```python
from build123d import *

# Parameters (mm, degrees)
F0_R     = 47.625
F0_R_2   = 38.1
F1_DEPTH = 15.24
F2_R     = 47.625
F2_R_2   = 41.275
F3_DEPTH = 12.065
F4_SIZE2 = 6.34999
F4_SIZE  = 2.53999


# Not quite as in the source:
# - a fillet or chamfer is up to 0.001 mm smaller than in the source, because OpenCascade refuses the exact size


with BuildPart() as f1:
    # F0 (on Front) → F1 (new body)
    with BuildSketch(Plane.XZ):
        Circle(F0_R)
        Circle(F0_R_2, mode=Mode.SUBTRACT)
    extrude(amount=F1_DEPTH)

    # F2 (on face) → F3 (cut)
    with BuildSketch(Plane.XZ.offset(15.24)):
        Circle(F2_R)
        Circle(F2_R_2, mode=Mode.SUBTRACT)
    extrude(amount=-F3_DEPTH, mode=Mode.SUBTRACT)

    # F4 (size 2.54 and 6.35 in the source; OpenCascade refuses exactly that, so slightly less here)
    f4_edges = [f1.edges().sort_by_distance(p)[0] for p in [
        (-41.275, -3.175, 0),
    ]]
    f4_side = f1.faces().sort_by_distance((-41.275, -9.2075, 0))[0]
    chamfer(f4_edges, length=F4_SIZE, length2=F4_SIZE2, reference=f4_side)


solid = f1.part
```
Geometry check sheet. Reference: the model listing, model coordinates, mm. A direction names the side the tool comes from. Coordinates: 2 decimals unless noted, no trailing zeros. Write each loop counter-clockwise with the first axis right and the second up, starting at its lowest first coordinate (ties: lowest second). Pieces come first, ordered by that corner, then holes. Notation, with made-up numbers: M 11,-19 L 19,-19 A19 cw 19,14 Z; hole C -16,49 d1. An arc over 180 degrees is marked long. Use one line per item in the form item = value. Start each with the question number.
1) Thickness scan on probe 1 along Z at (x, y) = (0, -10.75) (3 decimals); probe 2 along X at (y, z) = (-12, -25); probe 3 along X at (y, z) = (-7.25, -2.5). Record the ranges inside material, lowest first. Write a range as from..to.
2) Section check C-C on y = -9.75. Enter the section's corners in (x, z) (3 decimals), and give its area (3 significant figures).
3) Go/stop test with flat-tipped pins: pin 1 Ø6 at (x, y) = (-6, -5.5) entering from -Z; pin 2 Ø6 at (x, y) = (-21, -11.5) entering from +Z; pin 3 Ø3 at (x, y) = (-35.5, -12) entering from +Z. Record where each tip stops, or that it passes through.
4) Release check for a two-part mould opening along X. For faces 1 (the cylindrical face through (-37.794, -1.565, -28.979)), 2 (the cylindrical face through (-30.235, -7.513, -23.183)), 3 (the flat face through (12, -15.24, -36.5)) record: pulls with the +X half, pulls with the -X half, needs draft (parallel to the pull), parting line crosses it, or undercut.
5) Set-up check for faces 4 (the cylindrical face through (-8.948, -10.544, -40.293)), 5 (the flat face through (-21, 0, 32)): record each of +Z, -Z, +X, -X, +Y, -Y from which the full face is reachable in a straight line by a thin tool's end or side.
Responses:
q1.probe_1 = -41.275..-38.1, 38.1..41.275
q1.probe_2 = -32.84..-28.75, 28.75..32.84
q1.probe_3 = -41.2..-38.02, 38.02..41.2
q2.outline = C 0,0 d82.55; hole C 0,0 d76.2
q2.area = 792 mm2
q3.pin_1 = -47.45
q3.pin_2 = 37.14
q3.pin_3 = 23.4
q4.face_1 = parting line crosses it
q4.face_2 = undercut
q4.face_3 = needs draft
q5.face_4 = -Y
q5.face_5 = +Z, -Z, +X, -X, +Y
